Work out the finished part from the listing and answer in its coordinate system (mm). Face numbers are marked on the shaded views. A direction names the side the tool comes from. Round coordinates to 2 decimals unless told otherwise and drop trailing zeros. Loops run counter-clockwise (first coordinate to the right, second up) from the corner with the lowest first, then second, coordinate; pieces in that order, holes last.
```python
from build123d import *

# Parameters (mm, degrees)
RESSALTO_EXTRUS_O1_DEPTH   = 34
RESSALTO_EXTRUS_O1_2_DEPTH = 34
RESSALTO_EXTRUS_O2_DEPTH   = 2
RESSALTO_EXTRUS_O3_START   = 34
RESSALTO_EXTRUS_O3_DEPTH   = 2
CORTE_EXTRUS_O2_DEPTH      = 42


with BuildPart() as part:
    # Esbo_o1 → Ressalto-extrus_o1 (new body)
    with BuildSketch(Plane.XY):
        Polygon((76.215295477, -184), (184, -76.215295477), (184, 76.215295477), (76.215295477, 184), (-76.215295477, 184), (-184, 76.215295477), (-184, -76.215295477), (-76.215295477, -184), align=None)
        Polygon((180, -74.558441227), (180, 74.558441227), (74.558441227, 180), (-74.558441227, 180), (-180, 74.558441227), (-180, -74.558441227), (-74.558441227, -180), (74.558441227, -180), align=None, mode=Mode.SUBTRACT)
    extrude(amount=RESSALTO_EXTRUS_O1_DEPTH)



with BuildPart() as body_2:
    # Esbo_o1 → Ressalto-extrus_o1 2 (new body)
    with BuildSketch(Plane.XY):
        Polygon((62.132034356, -150), (150, -62.132034356), (150, 62.132034356), (62.132034356, 150), (-62.132034356, 150), (-150, 62.132034356), (-150, -62.132034356), (-62.132034356, -150), align=None)
        Polygon((146, -60.475180106), (146, 60.475180106), (60.475180106, 146), (-60.475180106, 146), (-146, 60.475180106), (-146, -60.475180106), (-60.475180106, -146), (60.475180106, -146), align=None, mode=Mode.SUBTRACT)
    extrude(amount=RESSALTO_EXTRUS_O1_2_DEPTH)


with BuildPart() as part_1:
    add(part.part)

    add(body_2.part)  # Ressalto-extrus_o2 merges body 2
    # Esbo_o1_3 → Ressalto-extrus_o2 (add)
    with BuildSketch(Plane.XY):
        Polygon((74.558441227, -180), (180, -74.558441227), (180, 74.558441227), (74.558441227, 180), (-74.558441227, 180), (-180, 74.558441227), (-180, -74.558441227), (-74.558441227, -180), align=None)
        Polygon((150, -62.132034356), (150, 62.132034356), (62.132034356, 150), (-62.132034356, 150), (-150, 62.132034356), (-150, -62.132034356), (-62.132034356, -150), (62.132034356, -150), align=None, mode=Mode.SUBTRACT)
    extrude(amount=RESSALTO_EXTRUS_O2_DEPTH)

    # Esbo_o1_4 → Ressalto-extrus_o3 (add)
    with BuildSketch(Plane.XY.offset(RESSALTO_EXTRUS_O3_START)):
        Polygon((74.558441227, -180), (180, -74.558441227), (180, 74.558441227), (74.558441227, 180), (-74.558441227, 180), (-180, 74.558441227), (-180, -74.558441227), (-74.558441227, -180), align=None)
        Polygon((150, -62.132034356), (150, 62.132034356), (62.132034356, 150), (-62.132034356, 150), (-150, 62.132034356), (-150, -62.132034356), (-62.132034356, -150), (62.132034356, -150), align=None, mode=Mode.SUBTRACT)
    extrude(amount=-RESSALTO_EXTRUS_O3_DEPTH)

    # Esbo_o5 → Corte-extrus_o2 (cut)
    with BuildSketch(Plane.XY.offset(34)):
        Polygon((-42.132034356, -146), (-57.872149726, -184), (76.215295477, -184), (184, -76.215295477), (184, 76.215295477), (76.215295477, 184), (-76.215295477, 184), (-184, 76.215295477), (-184, -76.215295477), (-89.185858225, -171.029437252), (-73.445742855, -133.029437252), (-146, -60.475180106), (-146, 60.475180106), (-60.475180106, 146), (60.475180106, 146), (146, 60.475180106), (146, -60.475180106), (60.475180106, -146), align=None)
    extrude(amount=-CORTE_EXTRUS_O2_DEPTH, mode=Mode.SUBTRACT)


solid = part_1.part
```
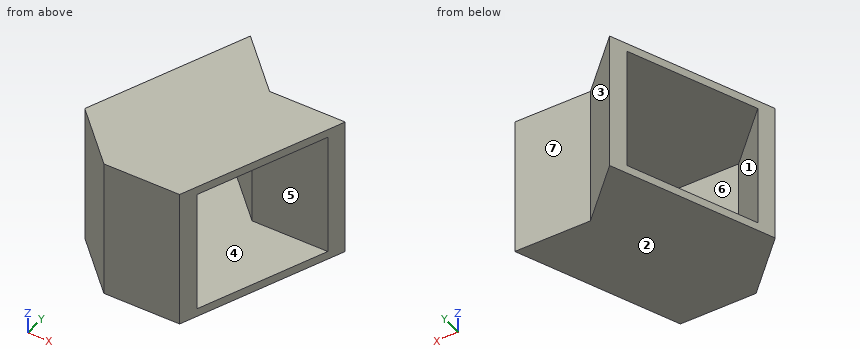
1. Find section A-A (z = 10). Write down the section's boundary in (x, y), then the cut area to 3 significant figures.
Answer key:
outline: (-89.19, -171.03) - (-76.22, -184) - (-57.87, -184) - (-56.22, -180) - (-74.56, -180) - (-87.53, -167.03) - close; (-75.1, -137.03) - (-62.13, -150) - (-43.79, -150) - (-42.13, -146) - (-60.48, -146) - (-73.45, -133.03) - close
area: 293 mm2
2. Determine the mould class of the marked faces 1, 2 and 3 for opening direction Z: +Z half, -Z half, draft (parallel to the pull), parting line (faces both ways), or undercut.
Answer key:
face 1: undercut
face 2: -Z half
face 3: draft
3. Given pin 1 (20 mm diameter, centred on x = -52, z = 13, fed in from +Y); pin 2 (6 mm diameter, centred on y = -165.5, z = 24.5, fed in from +X); pin 3 (8 mm diameter, centred on y = -176.5, z = 13, fed in from +X), each flat-ended and moving along its own axis, determine where each tip first touches the part or whether it passes through.
Answer key:
pin 1: stops at y = -144.48
pin 2: stops at x = -86.06
pin 3: stops at x = -56.22
4. Which of the six approach directions +Z, -Z, +X, -X, +Y, -Y give full straight-line access (tool end or side, diameter ignored) to the marked faces 4, 5, 6 and 7?
Answer key:
face 4: none
face 5: +X, -X
face 6: +X
face 7: +Z, -Z, +X, +Y
5. Find section D-D (x = -53). Write down the section's boundary in (y, z).
Answer key:
outline: (-172.24, 0) - (-146, 0) - (-146, 34) - (-172.24, 34) - (-172.24, 32) - (-150, 32) - (-150, 2) - (-172.24, 2) - close
6. Find section B-B (x = -66). Write down the section's boundary in (y, z).
Answer key:
outline: (-184, 0) - (-140.48, 0) - (-140.48, 34) - (-184, 34) - close; hole (-180, 2) - (-146.13, 2) - (-146.13, 32) - (-180, 32) - close
7. Find section C-C (y = -141). Write down the section's boundary in (x, z).
Answer key:
outline: (-76.75, 0) - (-65.48, 0) - (-65.48, 34) - (-76.75, 34) - (-76.75, 32) - (-71.13, 32) - (-71.13, 2) - (-76.75, 2) - close
8. Consider probe 1 along Z at (x, y) = (-76, -162); probe 2 along Y at (x, z) = (-45, 23); probe 3 along Y at (x, z) = (-65.5, 30.5). Determine where each line is inside the solid, lowest interval first.
Answer key:
probe 1: z = 0 to 2, 32 to 34
probe 2: y = -150 to -146
probe 3: y = -184 to -180, -146.63 to -140.98
